from build123d import *

# Parameters (mm, degrees)
SKETCH1_W          = 3
SKETCH1_H          = 20
BASE_EXTRUDE_DEPTH = 3


with BuildPart() as part:
    # Sketch1 → Base-Extrude (new body)
    with BuildSketch(Plane.XY):
        with BuildLine():
            Line((-720.928496368, -130.234955171), (-721.834448628, -88.561920568))
            ThreePointArc((-721.834448628, -88.561920568), (-713.861531309, -83.622429775), (-705.707617137, -88.257045566))
            ThreePointArc((-705.707617137, -88.257045566), (-703.559840829, -111.460770875), (-714.312380099, -132.134636275))
            ThreePointArc((-714.312380099, -132.134636275), (-718.013875072, -132.555038268), (-720.928496368, -130.234955171))
        make_face()
        with Locations((-715.695158937, -108.450949368)):
            Rectangle(SKETCH1_W, SKETCH1_H, mode=Mode.SUBTRACT)
    extrude(amount=BASE_EXTRUDE_DEPTH)


solid = part.part
Work out the finished part from the listing and answer in its coordinate system (mm). A direction names the side the tool comes from. Round coordinates to 2 decimals unless told otherwise and drop trailing zeros. Order: outer loops, then holes, each group sorted by start corner. A loop starts at its lowest first (then second) coordinate and runs counter-clockwise, first axis right, second up. Notation, with made-up numbers: M -6,72.25 L 15,72.25 A27 cw 15,93.25 Z; hole C -1,48.25 d4. An arc over 180 degrees is marked long. One line per item, written item: value.
Q1. Find section C-C on x = -715. Write down the section's boundary in (y, z), then the cut area to 3 significant figures.
Derived:
outline: M -132.45,0 L -118.45,0 L -118.45,3 L -132.45,3 Z; M -98.45,0 L -83.71,0 L -83.71,3 L -98.45,3 Z
area: 86.2 mm²
Q2. For faces 1 (the face through (-716, -98.451, 1)), 2 (the face through (-712, -108, 3)), determine the directions among +Z, -Z, +X, -X, +Y, -Y from which every point of the face is accessible in a straight line to the end or side of a thin tool.
Derived:
face 1: +Z, -Z
face 2: +Z, +X, -X, +Y, -Y
Q3. Determine the mould class of faces 3 (the face through (-713.999, -83.626, 1.479)), 4 (the face through (-717.195, -109, 1)), 5 (the face through (-717.96, -132.57, 1.48)), 6 (the face through (-714.195, -109, 1)) for opening direction Y: released by +Y, released by -Y, zero draft, split by the parting line, or undercut.
Derived:
face 3: released by +Y
face 4: undercut
face 5: released by -Y
face 6: undercut
Q4. Find section B-B on y = -115. Write down the section's boundary in (x, z).
Derived:
outline: M -721.26,0 L -717.2,0 L -717.2,3 L -721.26,3 Z; M -714.2,0 L -704.42,0 L -704.42,3 L -714.2,3 Z
Q5. Find section D-D on y = -95.5. Write down the section's boundary in (x, z), then the cut area to 3 significant figures.
Derived:
outline: M -721.68,0 L -703.57,0 L -703.57,3 L -721.68,3 Z
area: 54.3 mm²
Q6. Find section A-A on z = 2.45. Write down the section's boundary in (x, y), then the cut area to 3 significant figures.
Derived:
outline: M -721.83,-88.56 L -720.93,-130.23 A4.87 ccw -714.31,-132.13 A41.31 ccw -705.71,-88.26 A9.19 ccw Z; hole M -717.2,-118.45 L -714.2,-118.45 L -714.2,-98.45 L -717.2,-98.45 Z
area: 690 mm²
Q7. Straight lines are drawn through the part: line 1 (Y direction, x = -715.5, z = 2.6); line 2 (Y direction, x = -714.5, z = 2.2); line 3 (X direction, y = -108.5, z = 2.6). For each, find the intervals that lie inside material, in ascending order.
Derived:
line 1: -132.6 to -118.45, -98.45 to -83.8
line 2: -132.23 to -118.45, -98.45 to -83.66
line 3: -721.4 to -717.2, -714.2 to -703.09
